Build history of the part. All positions in model axes, mm. Face numbers are marked on the shaded views. Coordinates: 2 decimals unless noted, no trailing zeros. Order: outer loops, then holes, each group sorted by start corner. A loop starts at its lowest first (then second) coordinate and runs counter-clockwise, first axis right, second up. Notation, with made-up numbers: M 67,-8 L 87,-8 A24 ccw 87,13 Z; hole C 32,51 d10. An arc over 180 degrees is marked long. Use a Markdown table: item, result. Add a question column.
from build123d import *

# Parameters (mm, degrees)
SKETCH_1_R          = 30
EXTRUDE_1_DEPTH     = 65
SKETCH_2_R          = 27.5
CUT_EXTRUDE_1_DEPTH = 5
CUT_EXTRUDE_START   = -57
SKETCH_3_R          = 27.5
CUT_EXTRUDE_2_DEPTH = 57


with BuildPart() as part:
    # 草图1 → 凸台-拉伸1 (new body)
    with BuildSketch(Plane(origin=(0, 0, 0), x_dir=(1, 0, 0), z_dir=(0, 1, 0))):
        with Locations(Location((0, 0, 0), (0, 0, 270))):
            Circle(SKETCH_1_R)
    extrude(amount=EXTRUDE_1_DEPTH)

    # 草图2 → 切除-拉伸1 (cut)
    with BuildSketch(Plane(origin=(0, 65, 0), x_dir=(1, 0, 0), z_dir=(0, 1, 0))):
        with Locations(Location((0, 0, 0), (0, 0, 270))):
            Circle(SKETCH_2_R)
    extrude(amount=-CUT_EXTRUDE_1_DEPTH, mode=Mode.SUBTRACT)

    # 草图3 → 切除-拉伸2 (cut)
    with BuildSketch(Plane.XZ.offset(CUT_EXTRUDE_START)):
        with Locations(Location((0, 0, 0), (0, 0, 90))):
            Circle(SKETCH_3_R)
    extrude(amount=CUT_EXTRUDE_2_DEPTH, mode=Mode.SUBTRACT)


solid = part.part
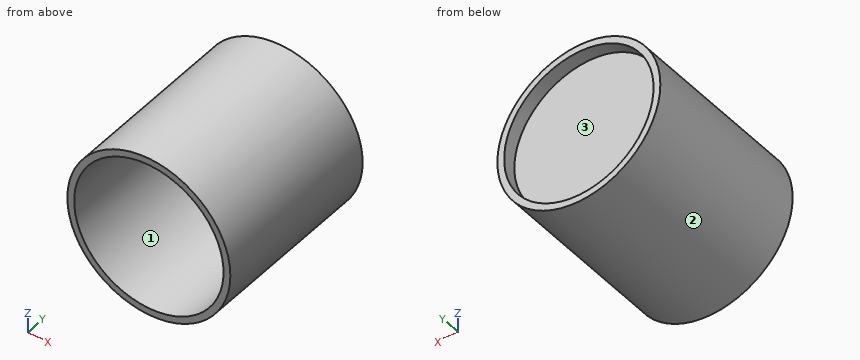
(1) Mould opens along Z. For the marked faces 1, 2 and 3 say: released by +Z, released by -Z, zero draft, split by the parting line, or undercut.
(2) Slice it at C-C on y = 55.5. Give the cut face in (x, z).
(3) Slice it at B-B on z = -12. Give the cut face in (x, y), and give its area (3 significant figures).
(4) Drill centre lines: line 1 along X through (y, z) = (23, 0); line 2 along Y through (x, z) = (24, -13); line 3 along Z through (x, y) = (18.5, 16.5). Where is each one in solid material? Low to high. Write a range as from..to.
(5) Slice it at A-A on x = 0. Give the cut face in (y, z), and give its area (3 significant figures).
(6) Drop flat-ended pins along their axis: P1, Ø8, axis at x = 8.5, y = 43, coming from the -Z side; P2, Ø2, axis at y = 54, z = 0.5, coming from the -X side; P3, Ø6, axis at x = -13, z = -18.5, coming from the -Y side. Give the stop position or say it passes through.
Solutions:
| question | item | result |
|---|---|---|
| 1 | face 1 | undercut |
| 1 | face 2 | split by the parting line |
| 1 | face 3 | undercut |
| 2 | outline | C 0,0 d60; hole C 0,0 d55 |
| 3 | outline | M -27.5,0 L -24.74,0 L -24.74,57 L 24.74,57 L 24.74,0 L 27.5,0 L 27.5,65 L 24.74,65 L 24.74,60 L -24.74,60 L -24.74,65 L -27.5,65 Z |
| 3 | area | 506 mm² |
| 4 | line 1 | -30..-27.5, 27.5..30 |
| 4 | line 2 | 57..60 |
| 4 | line 3 | -23.62..-20.35, 20.35..23.62 |
| 5 | outline | M 0,-30 L 65,-30 L 65,-27.5 L 60,-27.5 L 60,27.5 L 65,27.5 L 65,30 L 0,30 L 0,27.5 L 57,27.5 L 57,-27.5 L 0,-27.5 Z |
| 5 | area | 490 mm² |
| 6 | P1 | z = -29.66 |
| 6 | P2 | x = -30 |
| 6 | P3 | y = 57 |
